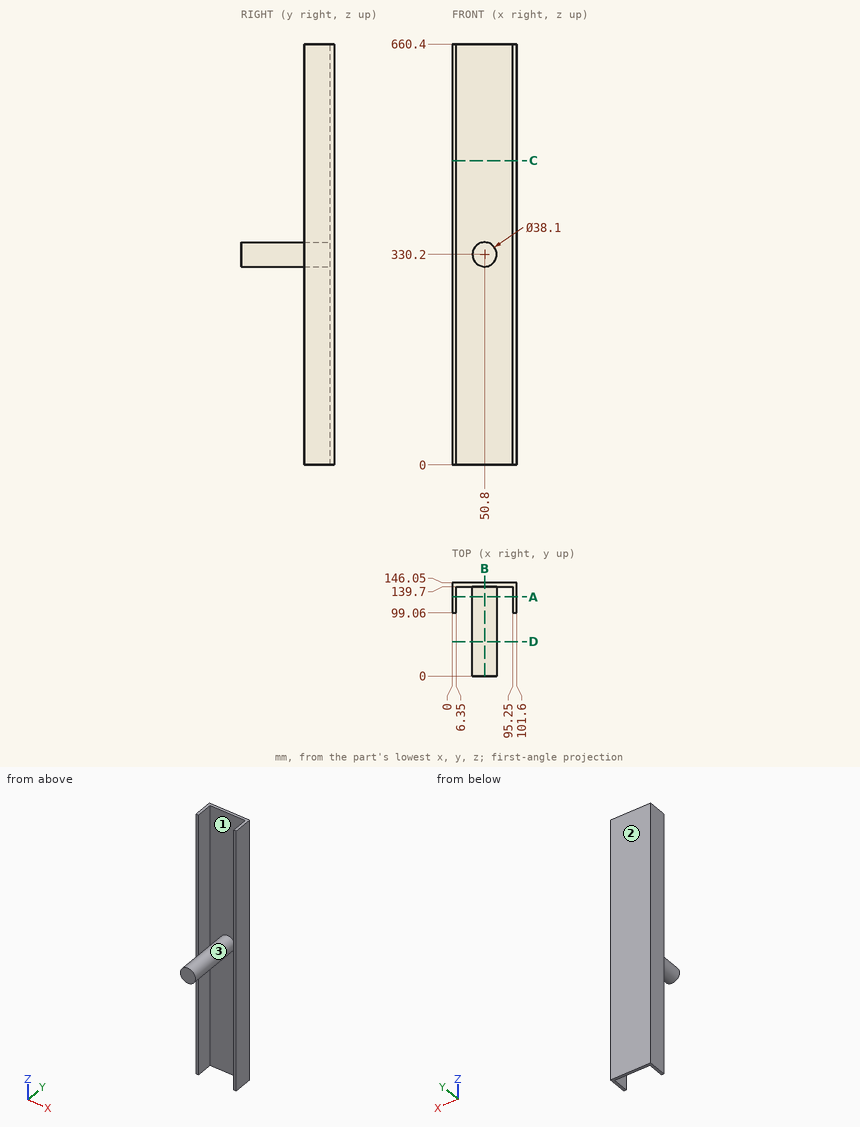
The figure shows three views and two pictorial views of one solid part (mm, origin at its lowest corner). Answer the questions. Give positions to 0.01 mm unless a question says otherwise; leave off trailing zeros. Loops run counter-clockwise (first coordinate to the right, second up) from the corner with the lowest first, then second, coordinate; pieces in that order, holes last. Notation, with made-up numbers: (78, 57) -> (104, 57) arc R15 cw to (104, 84) -> close; hole circle Ø9 at (8, 88). An arc over 180 degrees is marked (long way). Put each result on its own line as item: value. Start each with the question number.
Item 1: Each of these flat-tipped pins is pushed along its axis until it touches: P1, Ø7, axis at x = 98.5, z = 486, coming from the -Y side; P2, Ø1, axis at x = 54.5, y = 97.5, coming from the -Z side. Where does it stop, or does it pass through?
Item 2: Find the intervals of material crossed by L1, parallel to X at y = 138.5, z = 45; L2, parallel to Y at x = 79, z = 623; L3, parallel to Z at x = 51.5, y = 87, in increasing order. Write a range as [from, to].
Item 3: The part is cut by section D-D (y = 54). Give the vertices of the cut face in (x, z).
Item 4: The part is cut by section A-A (y = 124). Give the vertices of the cut face in (x, z).
Item 5: The part is cut by section C-C (z = 477.5). Give the vertices of the cut face in (x, y).
Item 6: The mould has two halves that part along X. Classify the marked faces 1, 2 and 3: released by +X, released by -X, zero draft, split by the parting line, or undercut.
Item 7: The part is cut by section B-B (x = 50.8). Give the vertices of the cut face in (y, z), then the cut area to 3 significant figures.
Answers below:
1. P1: y = 99.06
1. P2: z = 311.42
2. L1: [0, 6.35], [95.25, 101.6]
2. L2: [139.7, 146.05]
2. L3: [311.16, 349.24]
3. outline: circle Ø38.1 at (50.8, 330.2)
4. outline: (0, 0) -> (6.35, 0) -> (6.35, 660.4) -> (0, 660.4) -> close; circle Ø38.1 at (50.8, 330.2); (95.25, 0) -> (101.6, 0) -> (101.6, 660.4) -> (95.25, 660.4) -> close
5. outline: (0, 99.06) -> (6.35, 99.06) -> (6.35, 139.7) -> (95.25, 139.7) -> (95.25, 99.06) -> (101.6, 99.06) -> (101.6, 146.05) -> (0, 146.05) -> close
6. face 1: undercut
6. face 2: zero draft
6. face 3: undercut
7. outline: (0, 311.15) -> (139.7, 311.15) -> (139.7, 0) -> (146.05, 0) -> (146.05, 660.4) -> (139.7, 660.4) -> (139.7, 349.25) -> (0, 349.25) -> close
7. area: 9,520 mm2
